Part print with two shaded views. Sizes in mm from the minimum x, y, z corner. A direction names the side the tool comes from. Give positions to 0.01 mm unless a question says otherwise; leave off trailing zeros. Write each loop counter-clockwise with the first axis right and the second up, starting at its lowest first coordinate (ties: lowest second). Pieces come first, ordered by that corner, then holes. Notation, with made-up numbers: (27.25, 37.5) -> (61.25, 37.5) arc R28 ccw to (61.25, 73.5) -> close; hole circle Ø2 at (40.5, 66.5). An arc over 180 degrees is marked (long way). Answer as a JSON object with one key per item and string values.
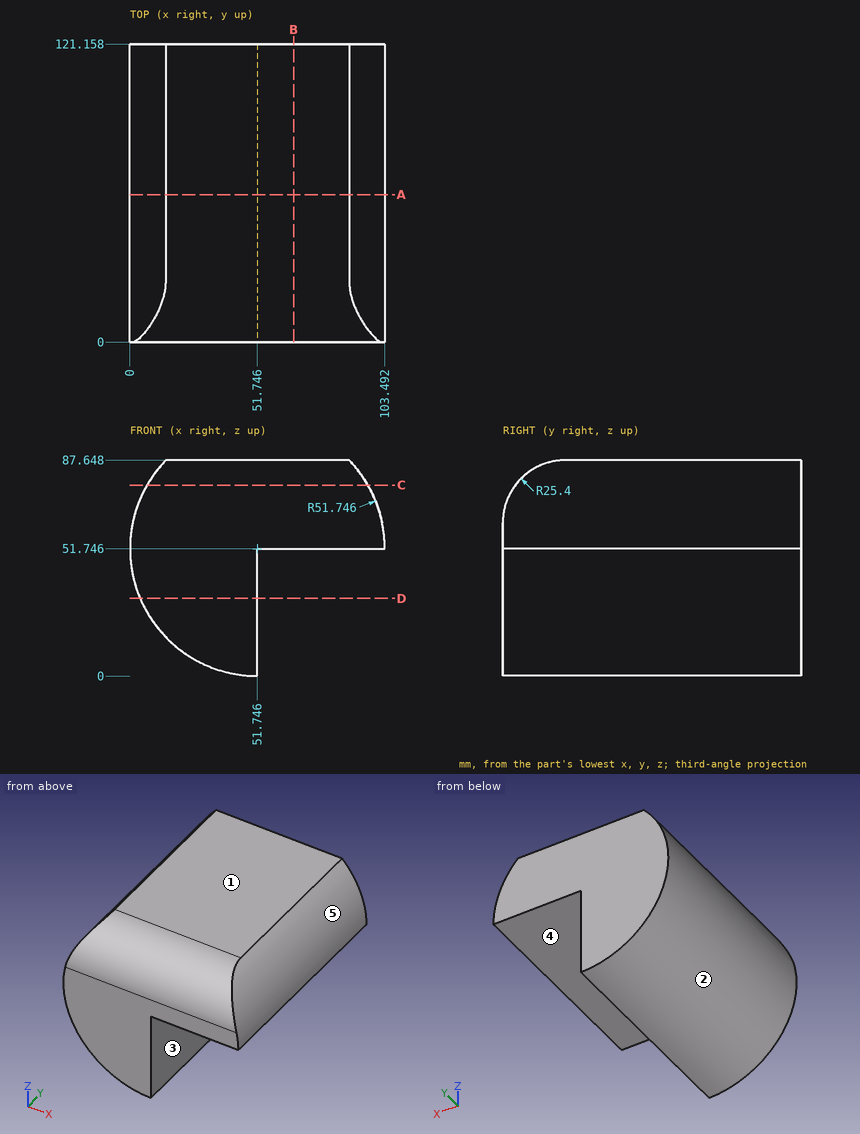
1) Pin check, flat tips, straight feed: pin 1 (5 mm diameter, centred on x = 43.5, y = 82.5, fed in from -Z); pin 2 (6 mm diameter, centred on x = 88.5, y = 98.5, fed in from -Z); pin 3 (8 mm diameter, centred on y = 71.5, z = 9, fed in from -X). Stop position of each tip, or through.
Model answer:
{"pin 1": "stops at z = 0.32", "pin 2": "stops at z = 51.75", "pin 3": "stops at x = 17.45"}
2) 3-axis set-ups, long thin cutter, end or side, ignore diameter. For the marked faces 4 and 5: which of +Z, -Z, +X, -X, +Y, -Y reach the whole face in a straight line?
Model answer:
{"face 4": "-Z, +X, +Y, -Y", "face 5": "+Z, +X, +Y, -Y"}
3) Slice it at A-A (y = 60). List the corners of the cut face in (x, z), then the cut area to 3 significant figures.
Model answer:
{"outline": "(14.48, 87.65) arc R51.75 ccw to (51.75, 0) -> (51.75, 51.75) -> (103.49, 51.75) arc R51.75 ccw to (89.01, 87.65) -> close", "area": "5,490 mm2"}
4) Slice it at D-D (z = 31.5). List the corners of the cut face in (x, y) (1 decimal), then the cut area to 3 significant figures.
Model answer:
{"outline": "(4.1, 0) -> (51.7, 0) -> (51.7, 121.2) -> (4.1, 121.2) -> close", "area": "5,770 mm2"}
5) Mould opens along X. For the marked faces 1, 2 and 3 say: released by +X, released by -X, zero draft, split by the parting line, or undercut.
Model answer:
{"face 1": "zero draft", "face 2": "released by -X", "face 3": "released by +X"}
6) Slice it at C-C (z = 77.5). List the corners of the cut face in (x, y), then the cut area to 3 significant figures.
Model answer:
{"outline": "(6.86, 5.09) -> (96.63, 5.09) -> (96.63, 121.16) -> (6.86, 121.16) -> close", "area": "10,400 mm2"}
7) Slice it at B-B (x = 66.5). List the corners of the cut face in (y, z).
Model answer:
{"outline": "(0, 51.75) -> (121.16, 51.75) -> (121.16, 87.65) -> (25.4, 87.65) arc R25.4 ccw to (0, 62.25) -> close"}
8) Wall check: probe 1 along Z at (x, y) = (89, 90) (1 decimal); probe 2 along X at (y, z) = (67.5, 72); probe 3 along Z at (x, y) = (14, 85). Give the ranges that are in metal, low to high.
Model answer:
{"probe 1": "z = 51.7 to 87.6", "probe 2": "x = 4.13 to 99.36", "probe 3": "z = 16.35 to 87.14"}
